Geometry check sheet. Reference: the model listing, model coordinates, mm. A direction names the side the tool comes from. Coordinates: 2 decimals unless noted, no trailing zeros. Loops run counter-clockwise (first coordinate to the right, second up) from the corner with the lowest first, then second, coordinate; pieces in that order, holes last.
from build123d import *

# Parameters (mm, degrees)
SKETCH_3_R             = 0.6225
SKETCH_3_R_2           = 5.25
CUT_EXTRUDE_1_DEPTH    = 10
EXTRUDE_START          = -1
SKETCH_4_R             = 12.5
SKETCH_4_R_2           = 8.75
EXTRUDE_1_DEPTH        = 1
SKETCH_9_R             = 0.6225
CUT_EXTRUDE_2_DEPTH    = 23.612164868
SKETCH_10_R            = 12.5
CUT_EXTRUDE_1339_DEPTH = 23.612164868
CHAMFER_1434_SIZE      = 0.5


with BuildPart() as part:
    # Эскиз1 → Повернуть1 (revolve)
    with BuildSketch(Plane(origin=(0, 0, 0), x_dir=(1, 0, 0), z_dir=(0, 1, 0))):
        Polygon((8.75, 1), (0, 1), (0, 0), (9.75, 0), (9.75, 15.1), (8.75, 15.1), align=None)
    revolve(axis=Axis((0, 0, 0), (0, 0, -1)))

    # Эскиз3 → Вырез-Вытянуть1 (cut)
    with BuildSketch(Plane.XY):
        with Locations((-4, 0)):
            Circle(SKETCH_3_R)
        with Locations((0, -4.75)):
            Circle(SKETCH_3_R)
        with Locations((3.96157844, 0)):
            Circle(SKETCH_3_R)
        with Locations((0, 4.75)):
            Circle(SKETCH_3_R)
        with Locations((7.601397898, -7.601397898)):
            Circle(SKETCH_3_R_2)
        with Locations((-7.601397898, -7.601397898)):
            Circle(SKETCH_3_R_2)
        with Locations((-7.601397898, 7.601397898)):
            Circle(SKETCH_3_R_2)
        with Locations((7.601397898, 7.601397898)):
            Circle(SKETCH_3_R_2)
    extrude(amount=-CUT_EXTRUDE_1_DEPTH, mode=Mode.SUBTRACT)

    # Эскиз4 → Бобышка-Вытянуть1 (add)
    with BuildSketch(Plane(origin=(0, 0, -15.1), x_dir=(-1, 0, 0), z_dir=(0, 0, -1)).offset(EXTRUDE_START)):
        Circle(SKETCH_4_R)
        with Locations(Location((0, 0, 0), (0, 0, 180))):
            Circle(SKETCH_4_R_2, mode=Mode.SUBTRACT)
    extrude(amount=EXTRUDE_1_DEPTH)

    # Эскиз9 → Вырез-Вытянуть2 (cut, through all)
    with BuildSketch(Plane.XY.offset(-14.1)):
        with Locations((7.866562941, 7.866562941)):
            Circle(SKETCH_9_R)
        with Locations((7.866562941, -7.866562941)):
            Circle(SKETCH_9_R)
        with Locations((-7.866562941, -7.866562941)):
            Circle(SKETCH_9_R)
        with Locations((-7.866562941, 7.866562941)):
            Circle(SKETCH_9_R)
    extrude(amount=-CUT_EXTRUDE_2_DEPTH, mode=Mode.SUBTRACT)

    # Эскиз10 → Cut-Extrude 1339 (cut, through all)
    with BuildSketch(Plane.XY.offset(-14.1)):
        with Locations((0, -22.4)):
            Circle(SKETCH_10_R)
    extrude(amount=-CUT_EXTRUDE_1339_DEPTH, mode=Mode.SUBTRACT)

    # Chamfer 1434
    chamfer_1434_edges = [part.edges().sort_by_distance(p)[0] for p in [
        (0, -9.9, -15.1),
    ]]
    chamfer(chamfer_1434_edges, length=CHAMFER_1434_SIZE)


solid = part.part
(1) Sectioned sample at D-D on x = 8. Record the cut outline in (y, z).
Findings:
outline: (-9.6, -15.1) - (-8.47, -15.1) - (-8.47, -14.1) - (-9.6, -14.1) - close; (-7.26, -15.1) - (-3.54, -15.1) - (-3.54, -10) - (-5.57, -10) - (-5.57, -14.1) - (-7.26, -14.1) - close; (-2.37, -1) - (2.37, -1) - (2.37, 0) - (-2.37, 0) - close; (3.54, -15.1) - (7.26, -15.1) - (7.26, -14.1) - (5.57, -14.1) - (5.57, -10) - (3.54, -10) - close; (8.47, -15.1) - (9.6, -15.1) - (9.6, -14.1) - (8.47, -14.1) - close
(2) Scan lines: L1, parallel to Y at x = 0, z = -0.35; L2, parallel to Z at x = -0.25, y = 6; L3, parallel to Y at x = 0, z = -11.5. Record each from-to range of solid material in increasing order.
Findings:
L1: y = -9.75 to -5.37, -4.13 to 4.13, 5.37 to 9.75
L2: z = -1 to 0
L3: y = -9.75 to -8.75, 8.75 to 9.75
(3) Gauge pin test, flat ends, axial feed: pin 1 Ø1.1 at (x, y) = (-7.87, -7.87) entering from -Z; pin 2 Ø1.5 at (y, z) = (1, -13.5) entering from +X; pin 3 Ø2 at (x, y) = (-4.5, 6.5) entering from +Z; pin 4 Ø14 at (x, y) = (0, 1.5) entering from -Z. Record the tip position at first contact, or that the pin passes through.
Findings:
pin 1: passes through
pin 2: stops at x = 12.49
pin 3: stops at z = -10
pin 4: stops at z = -1
(4) Access from +Z, -Z, +X, -X, +Y, -Y to the whole of each face (thin tool, end or side, straight path). Record for faces 1 (the cylindrical face through (3.91, -3.87, -0.53)), 2 (the cylindrical face through (-8.74, -0.38, -9.52)), 3 (the flat face through (0, 9, -15.1)).
Findings:
face 1: +Z
face 2: -Z
face 3: -Z, +X, -X, +Y, -Y
(5) Sectioned sample at A-A on x = 0. Record the cut outline in (y, z), and give its area (3 significant figures).
Findings:
outline: (-9.9, -14.6) - (-9.4, -15.1) - (-8.75, -15.1) - (-8.75, -1) - (-5.37, -1) - (-5.37, 0) - (-9.75, 0) - (-9.75, -14.1) - (-9.9, -14.1) - close; (-4.13, -1) - (4.13, -1) - (4.13, 0) - (-4.13, 0) - close; (5.37, -1) - (8.75, -1) - (8.75, -15.1) - (12.5, -15.1) - (12.5, -14.1) - (9.75, -14.1) - (9.75, 0) - (5.37, 0) - close
area: 48.0 mm2
(6) Sectioned sample at C-C on z = -6. Record the cut outline in (x, y), and give its area (3 significant figures).
Findings:
outline: (-9.38, -2.66) arc R5.25 cw to (-8.41, -2.41) arc R8.75 cw to (-8.41, 2.41) arc R5.25 cw to (-9.38, 2.66) arc R9.75 ccw to start; (-2.66, -9.38) arc R9.75 ccw to (2.66, -9.38) arc R5.25 cw to (2.41, -8.41) arc R8.75 cw to (-2.41, -8.41) arc R5.25 cw to start; (-2.66, 9.38) arc R5.25 cw to (-2.41, 8.41) arc R8.75 cw to (2.41, 8.41) arc R5.25 cw to (2.66, 9.38) arc R9.75 ccw to start; (8.41, -2.41) arc R5.25 cw to (9.38, -2.66) arc R9.75 ccw to (9.38, 2.66) arc R5.25 cw to (8.41, 2.41) arc R8.75 cw to start
area: 20.4 mm2
(7) Draft check along X on faces 4 (the cylindrical face through (-9.74, -0.43, -8.72)), 5 (the cylindrical face through (3.87, 3.91, -0.53)), 6 (the flat face through (0, 0, 0)). Enter one of: +X half, -X half, draft (parallel to the pull), parting line (faces both ways), or undercut.
Findings:
face 4: parting line
face 5: undercut
face 6: draft
(8) Sectioned sample at B-B on y = -6. Record the cut outline in (x, z), and give its area (3 significant figures).
Findings:
outline: (-10.97, -15.1) - (-6.37, -15.1) - (-6.37, -10) - (-7.69, -10) - (-7.69, -14.1) - (-10.97, -14.1) - close; (-2.6, -1) - (2.6, -1) - (2.6, 0) - (-2.6, 0) - close; (6.37, -15.1) - (10.97, -15.1) - (10.97, -14.1) - (7.69, -14.1) - (7.69, -10) - (6.37, -10) - close
area: 25.2 mm2
